Model file for the job. Use its own axes, mm. Coordinates: 2 decimals unless noted, no trailing zeros. Order: outer loops, then holes, each group sorted by start corner. A loop starts at its lowest first (then second) coordinate and runs counter-clockwise, first axis right, second up.
from build123d import *

# Parameters (mm, degrees)
SKETCH1_R           = 1.5
BOSS_EXTRUDE1_DEPTH = 3


with BuildPart() as part:
    # Sketch1 → Boss-Extrude1 (new body)
    with BuildSketch(Plane(origin=(0, 0, 0), x_dir=(0, 0, -1), z_dir=(1, 0, 0))):
        with BuildLine():
            Line((81.277391257, 21), (81.277391257, 18))
            Line((81.277391257, 18), (78.277391257, 18))
            Line((78.277391257, 18), (78.277391257, 8))
            Line((78.277391257, 8), (81.277391257, 8))
            Line((81.277391257, 8), (81.277391257, 0))
            Line((81.277391257, 0), (71.277391257, 0))
            Line((71.277391257, 0), (71.277391257, -3))
            Line((71.277391257, -3), (61.277391257, -3))
            Line((61.277391257, -3), (61.277391257, 0))
            Line((61.277391257, 0), (51.277391257, 0))
            Line((51.277391257, 0), (51.277391257, -3))
            Line((51.277391257, -3), (41.277391257, -3))
            Line((41.277391257, -3), (41.277391257, 0))
            Line((41.277391257, 0), (31.277391257, 0))
            Line((31.277391257, 0), (31.277391257, -3))
            Line((31.277391257, -3), (21.277391257, -3))
            Line((21.277391257, -3), (21.277391257, 0))
            Line((21.277391257, 0), (11.277391257, 0))
            Line((11.277391257, 0), (11.277391257, -3))
            Line((11.277391257, -3), (1.277391257, -3))
            Line((1.277391257, -3), (1.277391257, 0))
            Line((1.277391257, 0), (-8.722608743, 0))
            Line((-8.722608743, 0), (-8.722608743, 7))
            Line((-8.722608743, 7), (-2.722608743, 7))
            Line((-2.722608743, 7), (-2.722608743, 17))
            Line((-2.722608743, 17), (-8.722608743, 17))
            Line((-8.722608743, 17), (-8.722608743, 21))
            Line((-8.722608743, 21), (69.277391257, 21))
            Line((69.277391257, 21), (69.277391257, 27))
            ThreePointArc((69.277391257, 27), (75.277391257, 33), (81.277391257, 27))
            Line((81.277391257, 27), (81.277391257, 21))
        make_face()
        with Locations((75.277391257, 27)):
            Circle(SKETCH1_R, mode=Mode.SUBTRACT)
    extrude(amount=BOSS_EXTRUDE1_DEPTH)


solid = part.part
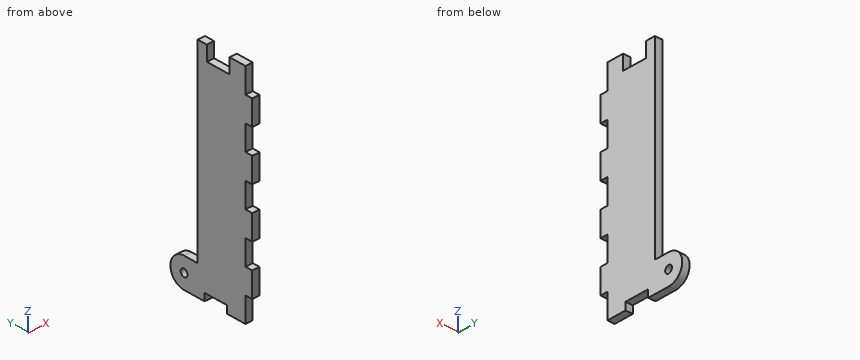
Q1. Drop flat-ended pins along their axis: P1, Ø1.5, axis at x = 1, y = 10.5, coming from the +Z side; P2, Ø1, axis at x = 1.5, z = -32.5, coming from the +Y side; P3, Ø0.9, axis at x = 2, y = -1.5, coming from the +Z side. Give the stop position or say it passes through.
Established:
P1: stops at z = 2.72
P2: stops at y = 21
P3: stops at z = -1.28
Q2. Cut at B-B, the plane z = -66.5. List the corners of the cut face in (x, y).
Established:
outline: (0, -3) - (3, -3) - (3, 21) - (0, 21) - close
Q3. Cut at A-A, the plane y = -1. List the corners of the cut face in (x, z).
Established:
outline: (0, -71.28) - (3, -71.28) - (3, -61.28) - (0, -61.28) - close; (0, -51.28) - (3, -51.28) - (3, -41.28) - (0, -41.28) - close; (0, -31.28) - (3, -31.28) - (3, -21.28) - (0, -21.28) - close; (0, -11.28) - (3, -11.28) - (3, -1.28) - (0, -1.28) - close
Q4. Probe line 1 (Z direction, x = 0.6, y = -0.5); line 2 (Y direction, x = 1.3, z = -46); line 3 (Z direction, x = 2.4, y = 28). List the from-to ranges inside material, lowest first.
Established:
line 1: z = -71.28 to -61.28, -51.28 to -41.28, -31.28 to -21.28, -11.28 to -1.28
line 2: y = -3 to 21
line 3: z = -81.19 to -76.4, -74.16 to -69.36
Q5. Cut at C-C, the plane y = 24. List the corners of the cut face in (x, z).
Established:
outline: (0, -81.28) - (3, -81.28) - (3, -69.28) - (0, -69.28) - close
